Can you work these out from the model? Positions are in its coordinate system, mm. A direction names the side the tool comes from. Round coordinates to 2 decimals unless told otherwise and drop trailing zeros. Loops run counter-clockwise (first coordinate to the right, second up) from the corner with the lowest first, then second, coordinate; pieces in that order, holes last.
Autodesk Inventor part; units mm, degrees
ref_plane "YZ Plane" through (0, 0, 0) normal (1, 0, 0) x (0, 1, 0)
ref_plane "XZ Plane" through (0, 0, 0) normal (0, 1, 0) x (-1, 0, 0)
ref_plane "XY Plane" through (0, 0, 0) normal (0, 0, 1) x (1, 0, 0)
sketch "スケッチ1" plane through (0, 0, 0) normal (0, 1, 0) x (-1, 0, 0)
  line L0 (85.0374, 519.8276) -> (82.0374, 519.8276)
  line L1 (82.0374, 519.8276) -> (82.0374, 369.8276)
  line L2 (82.0374, 369.8276) -> (85.0374, 369.8276)
  line L3 (85.0374, 369.8276) -> (85.0374, 519.8276)
  line L4 (160.0374, 372.8276) -> (85.0374, 372.8276)
  line L5 (85.0374, 372.8276) -> (85.0374, 369.8276)
  line L6 (85.0374, 369.8276) -> (160.0374, 369.8276)
  line L7 (160.0374, 369.8276) -> (160.0374, 372.8276)
  line L8 (163.0374, 372.8276) -> (160.0374, 372.8276)
  line L9 (160.0374, 372.8276) -> (160.0374, 222.8276)
  line L10 (160.0374, 222.8276) -> (163.0374, 222.8276)
  line L11 (163.0374, 222.8276) -> (163.0374, 372.8276)
  line L12 (160.0374, 225.8276) -> (85.0374, 225.8276)
  line L13 (85.0374, 225.8276) -> (85.0374, 222.8276)
  line L14 (85.0374, 222.8276) -> (160.0374, 222.8276)
  line L15 (160.0374, 222.8276) -> (160.0374, 225.8276)
  line L16 (85.0374, 225.8276) -> (82.0374, 225.8276)
  line L17 (82.0374, 225.8276) -> (82.0374, 75.8276)
  line L18 (82.0374, 75.8276) -> (85.0374, 75.8276)
  line L19 (85.0374, 75.8276) -> (85.0374, 225.8276)
  point P0 (0, 0)
  dimension "d0" = 150
  dimension "d1" = 3
  dimension "d2" = 3
  dimension "d3" = 75
  dimension "d4" = 3
  dimension "d5" = 150
  dimension "d6" = 75
  dimension "d7" = 3
  dimension "d8" = 3
  dimension "d9" = 150
extrude "押し出し1" add sketch "スケッチ1" along normal blind 70
sketch "スケッチ2" plane through (-82.0374, 0, 519.8276) normal (1, 0, 0) x (0, 0, -1)
  point P0 (519.8276, 0)
sketch "スケッチ3" plane through (0, 70, 0) normal (0, 1, 0) x (1, 0, 0)
  line L0 (-160.0374, -516.8276) -> (-85.0374, -516.8276)
  line L1 (-85.0374, -516.8276) -> (-85.0374, -519.8276)
  line L2 (-85.0374, -519.8276) -> (-160.0374, -519.8276)
  line L3 (-160.0374, -519.8276) -> (-160.0374, -516.8276)
  line L4 (-85.0374, -372.8276) -> (-85.0374, -519.8276)
  line L5 (-85.0374, -519.8276) -> (-82.0374, -519.8276)
  line L6 (-160.0374, -75.8276) -> (-85.0374, -75.8276)
  line L7 (-85.0374, -75.8276) -> (-85.0374, -78.8276)
  line L8 (-85.0374, -78.8276) -> (-160.0374, -78.8276)
  line L9 (-160.0374, -78.8276) -> (-160.0374, -75.8276)
  line L10 (-85.0374, -75.8276) -> (-85.0374, -222.8276)
  line L11 (-82.0374, -75.8276) -> (-85.0374, -75.8276)
  point P0 (0, 0)
  dimension "d12" = 75
  dimension "d13" = 3
  dimension "d14" = 75
  dimension "d15" = 3
extrude "押し出し2" add sketch "スケッチ3" against normal blind 70
properties part number "recreat2"
(1) We'd pull the mould along Z, two halves only. Please class faces 1 (the flat face through (-120, 35, 75.828)), 2 (the flat face through (-120, 35, 369.828)), 3 (the flat face through (-163.037, 35, 297)): released by +Z, released by -Z, zero draft, split by the parting line, or undercut.
(2) Suppose I cut it at C-C (z = 431). Write out the boundary of the cut face in (x, y), then the cut area to 3 significant figures.
(3) Which directions (+Z, -Z, +X, -X, +Y, -Y) give clear straight access to the entire face, cutting with the end or side of a thin tool? Please do faces 4 (the flat face through (-125, 35, 372.828)), 5 (the flat face through (-122, 35, 225.828)), 6 (the flat face through (-161, 0, 299)).
(4) For pin 1 (21 mm diameter, centred on y = 45.5, z = 281.5, fed in from +X); pin 2 (0.9 mm diameter, centred on y = 51.5, z = 77.5, fed in from -X); pin 3 (21 mm diameter, centred on y = 49.5, z = 151, fed in from -X), each with a flat end and sliding along its axis, tell me the tip position at first contact or that it passes through.
(5) Suppose I cut it at A-A (x = -114.5). Write out the boundary of the cut face in (y, z).
(6) Suppose I cut it at B-B (y = 52). Write out the boundary of the cut face in (x, z).
(7) If I drill on line 1 (Z direction, x = -129, y = 43); line 2 (X direction, y = 53, z = 467); line 3 (X direction, y = 8.5, z = 248.5), over which ranges is the centre line in solid material (lowest first)?
Check result:
1. face 1: released by -Z
1. face 2: undercut
1. face 3: zero draft
2. outline: (-85.04, 0) - (-82.04, 0) - (-82.04, 70) - (-85.04, 70) - close
2. area: 210 mm2
3. face 4: -X, +Y, -Y
3. face 5: +X, +Y, -Y
3. face 6: +Z, -Z, +X, -X, -Y
4. pin 1: stops at x = -160.04
4. pin 2: stops at x = -160.04
4. pin 3: stops at x = -85.04
5. outline: (0, 75.83) - (70, 75.83) - (70, 78.83) - (0, 78.83) - close; (0, 222.83) - (70, 222.83) - (70, 225.83) - (0, 225.83) - close; (0, 369.83) - (70, 369.83) - (70, 372.83) - (0, 372.83) - close; (0, 516.83) - (70, 516.83) - (70, 519.83) - (0, 519.83) - close
6. outline: (-163.04, 222.83) - (-85.04, 222.83) - (-85.04, 78.83) - (-160.04, 78.83) - (-160.04, 75.83) - (-82.04, 75.83) - (-82.04, 225.83) - (-160.04, 225.83) - (-160.04, 369.83) - (-82.04, 369.83) - (-82.04, 519.83) - (-160.04, 519.83) - (-160.04, 516.83) - (-85.04, 516.83) - (-85.04, 372.83) - (-163.04, 372.83) - close
7. line 1: z = 75.83 to 78.83, 222.83 to 225.83, 369.83 to 372.83, 516.83 to 519.83
7. line 2: x = -85.04 to -82.04
7. line 3: x = -163.04 to -160.04
